Input: dimensioned drawing with shaded views. Units: mm. Origin: part minimum x, y, z. A direction names the side the tool comes from. Give positions to 0.01 mm unless a question says otherwise; leave off trailing zeros. Loops run counter-clockwise (first coordinate to the right, second up) from the corner with the lowest first, then second, coordinate; pieces in that order, holes last. Notation, with made-up numbers: (-13.5, 49) -> (-1.5, 49) arc R18 ccw to (-1.5, 74) -> close; hole circle Ø10 at (69.5, 37). An arc over 180 degrees is marked (long way). Answer in a Markdown table with one row per item. Add a question column.
1) Draft query along X for the marked faces 3, 4 and 5. Return one class per face: +X half, -X half, draft (parallel to the pull), parting line (faces both ways), or undercut.
2) Section query A-A (y = 8). Give the number of separate pieces and of enclosed holes in the cut face, plus the area to 3 significant figures.
3) Section query D-D (z = 33). Return the cut outline in (x, y).
4) Line query: line 1 (X direction, y = 9, z = 52); line 2 (Z direction, x = 26, y = 30.5); line 3 (X direction, y = 13, z = 8). Output: solid intervals per line, ascending. Write a range as from..to.
5) Section query C-C (x = 22). Return the cut outline in (y, z), plus the area to 3 significant figures.
6) First-contact query: P1, Ø15.5, axis at x = 36.5, z = 52.5, coming from the +Y side; P2, Ø6, axis at x = 42, z = 63.5, coming from the +Y side. Flat tips, straight axial feed; report the tip coordinate or a pass-through.
7) Access query for the marked faces 1 and 2. Directions: +Z, -Z, +X, -X, +Y, -Y. A direction counts if a zero-diameter tool reaches every point of the face in a straight line with its end or side. Return the directions, or none.
8) Section query B-B (y = 26). Return the cut outline in (x, z).
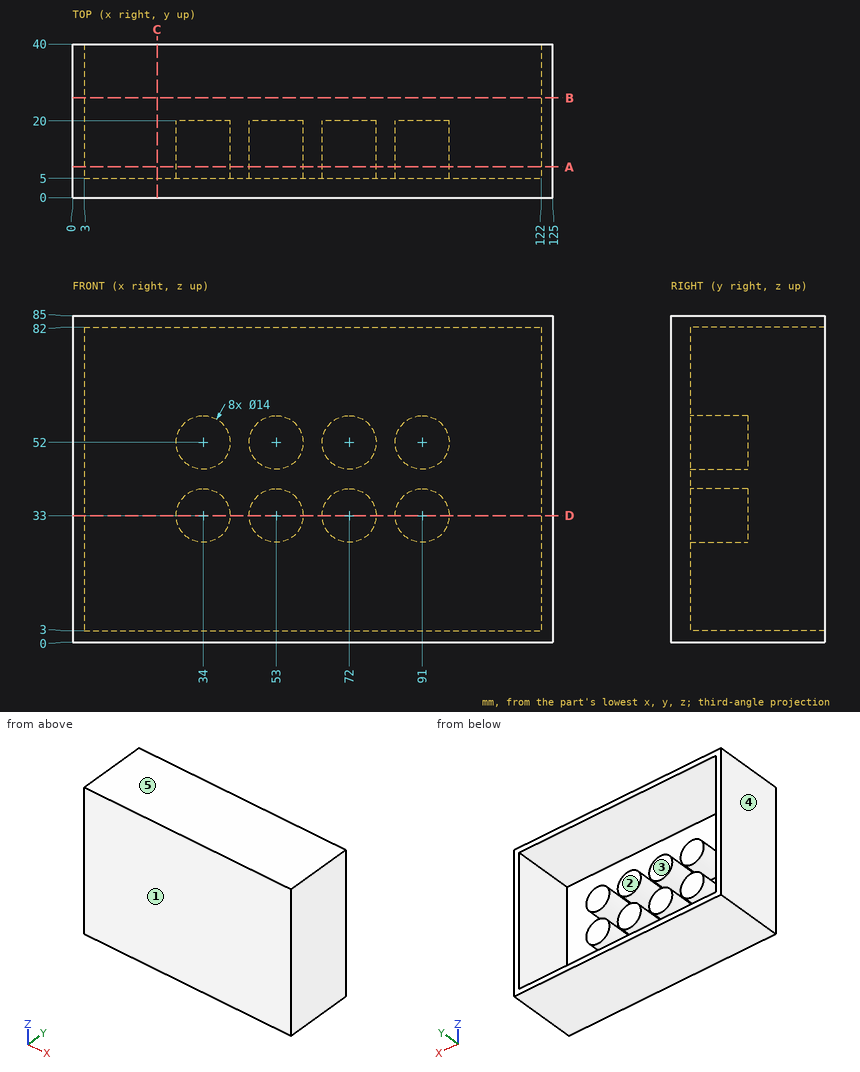
Evaluation:
| question | item | result |
|---|---|---|
| 1 | face 3 | undercut |
| 1 | face 4 | -X half |
| 1 | face 5 | draft |
| 2 | separate pieces | 9 |
| 2 | enclosed holes | 1 |
| 2 | area | 2,460 mm² |
| 3 | outline | (0, 0) -> (125, 0) -> (125, 40) -> (122, 40) -> (122, 5) -> (98, 5) -> (98, 20) -> (84, 20) -> (84, 5) -> (79, 5) -> (79, 20) -> (65, 20) -> (65, 5) -> (60, 5) -> (60, 20) -> (46, 20) -> (46, 5) -> (41, 5) -> (41, 20) -> (27, 20) -> (27, 5) -> (3, 5) -> (3, 40) -> (0, 40) -> close |
| 4 | line 1 | 0..3, 27..41, 46..60, 65..79, 84..98, 122..125 |
| 4 | line 2 | 0..3, 82..85 |
| 4 | line 3 | 0..3, 122..125 |
| 5 | outline | (0, 0) -> (40, 0) -> (40, 3) -> (5, 3) -> (5, 82) -> (40, 82) -> (40, 85) -> (0, 85) -> close |
| 5 | area | 635 mm² |
| 6 | P1 | y = 20 |
| 6 | P2 | y = 5 |
| 7 | face 1 | +Z, -Z, +X, -X, -Y |
| 7 | face 2 | +Y |
| 8 | outline | (0, 0) -> (125, 0) -> (125, 85) -> (0, 85) -> close; hole (3, 3) -> (122, 3) -> (122, 82) -> (3, 82) -> close |
